from build123d import *

# Parameters (mm, degrees)
SKETCH_1_R          = 2
EXTRUDE_1_DEPTH     = 3
EXTRUDE_2_DEPTH     = 6
SKETCH_3_R          = 1
CUT_EXTRUDE_1_DEPTH = 10


with BuildPart() as part:
    # 草图1 → 凸台-拉伸1 (new body)
    with BuildSketch(Plane.XY):
        Circle(SKETCH_1_R)
    extrude(amount=EXTRUDE_1_DEPTH)

    # 草图2 → 凸台-拉伸2 (add)
    with BuildSketch(Plane.XY.offset(3)):
        Polygon((1.760877545, 3.024782682), (-1.739099871, 3.037356028), (-3.499977416, 0.012573346), (-1.760877545, -3.024782682), (1.739099871, -3.037356028), (3.499977416, -0.012573346), align=None)
    extrude(amount=EXTRUDE_2_DEPTH)

    # 草图3 → 切除-拉伸1 (cut)
    with BuildSketch(Plane.XY.offset(9)):
        Circle(SKETCH_3_R)
    extrude(amount=-CUT_EXTRUDE_1_DEPTH, mode=Mode.SUBTRACT)


solid = part.part
Can you work these out from the model? Positions are in its coordinate system, mm. A direction names the side the tool comes from. Give positions to 0.01 mm unless a question says otherwise; leave off trailing zeros. Loops run counter-clockwise (first coordinate to the right, second up) from the corner with the lowest first, then second, coordinate; pieces in that order, holes last. Notation, with made-up numbers: (4.5, 84) -> (39.5, 84) arc R35 ccw to (39.5, 119) -> close; hole circle Ø2 at (-17.75, 81). An arc over 180 degrees is marked (long way). Write item = value, one per line.
1) Suppose I cut it at B-B on z = 5. Write out the boundary of the cut face in (x, y), then the cut area to 3 significant figures.
Check result:
outline = (-3.5, 0.01) -> (-1.76, -3.02) -> (1.74, -3.04) -> (3.5, -0.01) -> (1.76, 3.02) -> (-1.74, 3.04) -> close; hole circle Ø2 at (0, 0)
area = 28.7 mm2
2) Thinking about a two-plate mould opening in X: for faces 3 (the flat face through (1, -1, 0)), 4 (the flat face through (2.643, 1.485, 5.958)), 5 (the cylindrical face through (0, -1, 5)), which applies, released by +X, released by -X, zero draft, split by the parting line, or undercut?
Check result:
face_3 = zero draft
face_4 = released by +X
face_5 = undercut
3) For faces 1 (the flat face through (1, 1, 9)), 2 (the flat face through (2, 1, 3)), which set-ups out of +Z, -Z, +X, -X, +Y, -Y let a thin tool reach every point of the face, with its end or its side?
Check result:
face_1 = +Z, +X, -X, +Y, -Y
face_2 = -Z
4) I need wall thicknesses on L1, parallel to Y at x = 0, z = 2.25; L2, parallel to Z at x = -0.5, y = -2; L3, parallel to Y at x = 0, z = 5.75. Which ranges of each line are inside material? Lowest first, please. Write a range as from..to.
Check result:
L1 = -2..-1, 1..2
L2 = 3..9
L3 = -3.03..-1, 1..3.03
5) Suppose I cut it at C-C on x = 0. Write out the boundary of the cut face in (y, z).
Check result:
outline = (-3.03, 3) -> (-2, 3) -> (-2, 0) -> (-1, 0) -> (-1, 9) -> (-3.03, 9) -> close; (1, 0) -> (2, 0) -> (2, 3) -> (3.03, 3) -> (3.03, 9) -> (1, 9) -> close
6) Will these pins go through, and if not, where does the flat tip stop? pin 1 (1 mm diameter, centred on y = 1.5, z = 4.5, fed in from -X); pin 2 (2 mm diameter, centred on x = 1.5, z = 5.5, fed in from +Y); pin 3 (1.5 mm diameter, centred on y = 2.5, z = 6, fed in from -X).
Check result:
pin_1 = -2.93
pin_2 = 3.03
pin_3 = -2.49
7) Suppose I cut it at D-D on x = 1.5. Write out the boundary of the cut face in (y, z).
Check result:
outline = (-3.04, 3) -> (-1.32, 3) -> (-1.32, 0) -> (1.32, 0) -> (1.32, 3) -> (3.03, 3) -> (3.03, 9) -> (-3.04, 9) -> close
8) Suppose I cut it at A-A on y = 0.5. Write out the boundary of the cut face in (x, z), then the cut area to 3 significant figures.
Check result:
outline = (-3.22, 3) -> (-1.94, 3) -> (-1.94, 0) -> (-0.87, 0) -> (-0.87, 9) -> (-3.22, 9) -> close; (0.87, 0) -> (1.94, 0) -> (1.94, 3) -> (3.21, 3) -> (3.21, 9) -> (0.87, 9) -> close
area = 34.6 mm2
